```python
from build123d import *

# Parameters (mm, degrees)
F1_DEPTH = 304.8
F4_D     = 7.62
F4_DEPTH = 30.48
F4_TIP   = 2.2892789585
F5_D     = 7.62
F5_DEPTH = 30.48
F5_TIP   = 2.2892789585


with BuildPart() as f1:
    # F0 (on Front) → F1 (new body)
    with BuildSketch(Plane.XZ):
        Polygon((-39.024540448, 51.035306699), (-183.487040448, 51.035306699), (-183.487040448, -2.050693301), (-167.612040448, 7.1147422224), (-167.612040448, -31.9171288244), (-183.487040448, -22.751693301), (-183.487040448, -101.364693301), (-31.087040448, -101.364693301), (-31.087040448, 30.461306699), (-39.024540448, 30.461306699), align=None)
        Polygon((-23.149540448, 30.461306699), (-31.087040448, 30.461306699), (-31.087040448, -101.364693301), (121.312959552, -101.364693301), (121.312959552, -22.751693301), (105.437959552, -31.9171288244), (105.437959552, 7.1147422224), (121.312959552, -2.050693301), (121.312959552, 51.035306699), (-23.149540448, 51.035306699), align=None)
    extrude(amount=F1_DEPTH)

    # F4
    with Locations(Plane.YZ.offset(105.437959552)):
        with Locations((-63.5, -12.401193301), (-165.1, -12.401193301), (-266.7, -12.401193301)):
            Hole(F4_D / 2, depth=F4_DEPTH)
            with Locations((0, 0, -(F4_DEPTH + F4_TIP / 2))):  # 118° drill point
                Cone(0, F4_D / 2, F4_TIP, mode=Mode.SUBTRACT)

    # F5
    with Locations(Plane(origin=(-167.612040448, 0, 0), x_dir=(0, -1, 0), z_dir=(-1, 0, 0))):
        with Locations((63.5, -12.401193301), (165.1, -12.401193301), (266.7, -12.401193301)):
            Hole(F5_D / 2, depth=F5_DEPTH)
            with Locations((0, 0, -(F5_DEPTH + F5_TIP / 2))):  # 118° drill point
                Cone(0, F5_D / 2, F5_TIP, mode=Mode.SUBTRACT)


solid = f1.part
```
Geometry check sheet. Reference: the model listing, model coordinates, mm. A direction names the side the tool comes from. Give positions to 0.01 mm unless a question says otherwise; leave off trailing zeros. Loops run counter-clockwise (first coordinate to the right, second up) from the corner with the lowest first, then second, coordinate; pieces in that order, holes last. Notation, with made-up numbers: M 25.25,65 L 73.25,65 A14 ccw 73.25,91 Z; hole C -22,10 d7. An arc over 180 degrees is marked long. Write item = value, one per line. Start each with the question number.
1. Draft check along Y on faces 4 (the face through (-33, 0, -24)), 5 (the face through (-31, -150, 30.461)), 6 (the face through (-152.159, -263.066, -11.257)). Enter one of: +Y half, -Y half, draft (parallel to the pull), parting line (faces both ways), or undercut.
2. Section check A-A, the plane z = 37. Enter the section's corners in (x, y), plus the area to 3 significant figures.
3. Tool access check on faces 1 (the face through (89.985, -60.477, -14.72)), 2 (the face through (113.49, -150.27, -27.27)), 3 (the face through (-39.025, -150, 41)). Record the directions out of +Z, -Z, +X, -X, +Y, -Y that give a thin tool (end or side, any length) a straight path to the whole face; none if there is none.
4. Thickness scan on probe 1 along Z at (x, y) = (-144.5, -165.1); probe 2 along X at (y, z) = (-26, -31.5); probe 3 along X at (y, z) = (-66, -27.5). Record the ranges inside material, lowest first.
5. Go/stop test with flat-tipped pins: P1, Ø4.5, axis at y = -63.5, z = -12.4, coming from the -X side; P2, Ø2, axis at y = -195.5, z = -6.5, coming from the -X side; P3, Ø12, axis at y = -266.7, z = -12.4, coming from the +X side. Record where each tip stops, or that it passes through.
6. Section check B-B, the plane y = -154. Enter the section's corners in (x, z).
Values follow:
q1.face_4 = +Y half
q1.face_5 = draft
q1.face_6 = undercut
q2.outline = M -183.49,-304.8 L -39.02,-304.8 L -39.02,0 L -183.49,0 Z; M -23.15,-304.8 L 121.31,-304.8 L 121.31,0 L -23.15,0 Z
q2.area = 88,100 mm^2
q3.face_1 = +X
q3.face_2 = +Y, -Y
q3.face_3 = +Z, +Y, -Y
q4.probe_1 = -101.36 to -16.21, -8.59 to 51.04
q4.probe_2 = -183.49 to -168.33, -167.61 to 105.44, 106.16 to 121.31
q4.probe_3 = -183.49 to -175.26, -167.61 to 105.44, 113.09 to 121.31
q5.P1 = -136.2
q5.P2 = -167.61
q5.P3 = 105.44
q6.outline = M -183.49,-101.36 L 121.31,-101.36 L 121.31,-22.75 L 105.44,-31.92 L 105.44,7.11 L 121.31,-2.05 L 121.31,51.04 L -23.15,51.04 L -23.15,30.46 L -39.02,30.46 L -39.02,51.04 L -183.49,51.04 L -183.49,-2.05 L -167.61,7.11 L -167.61,-31.92 L -183.49,-22.75 Z
